Autodesk Inventor part; units mm, degrees
ref_plane "YZ Plane" through (0, 0, 0) normal (1, 0, 0) x (0, 1, 0)
ref_plane "XZ Plane" through (0, 0, 0) normal (0, 1, 0) x (-1, 0, 0)
ref_plane "XY Plane" through (0, 0, 0) normal (0, 0, 1) x (1, 0, 0)
sketch "Sketch1" plane through (0, 0, 0) normal (0, 0, 1) x (1, 0, 0)
  line L0 (0, 0) -> (861.06, 0)
  line L1 (861.06, 0) -> (861.06, 160.02)
  line L2 (861.06, 160.02) -> (0, 160.02)
  line L3 (0, 160.02) -> (0, 0)
  dimension "d2" = 861.06
  dimension "d3" = 160.02
extrude "Extrusion1" add sketch "Sketch1" along normal blind 4.7625
sketch "Sketch2" plane through (0, 0, 4.7625) normal (0, 0, 1) x (1, 0, 0)
  line L0 (849.63, 151.0147) -> (11.43, 151.0147)
  line L1 (887.73, 10.6797) -> (-26.67, 10.6797)
  line L2 (849.63, 848.8797) -> (849.63, 10.6797)
  line L3 (11.43, 848.8797) -> (11.43, 10.6797)
  line L4 (849.63, 10.6797) -> (11.43, 10.6797)
  line L5 (11.43, 10.6797) -> (11.43, 151.0147)
  line L6 (11.43, 151.0147) -> (849.63, 151.0147)
  line L7 (849.63, 151.0147) -> (849.63, 10.6797)
  point P0 (0, 0)
extrude "Extrusion2" add sketch "Sketch2" along normal blind 25.4
properties part number "gatorboard_01875in_front_door"
Work out the finished part from the listing and answer in its coordinate system (mm). A direction names the side the tool comes from. Give positions to 0.01 mm unless a question says otherwise; leave off trailing zeros. Loops run counter-clockwise (first coordinate to the right, second up) from the corner with the lowest first, then second, coordinate; pieces in that order, holes last. Notation, with made-up numbers: (-27.75, 69.25) - (-1.75, 69.25) arc R17 ccw to (-1.75, 97.25) - close; hole circle Ø5 at (-1, -30.75). An arc over 180 degrees is marked (long way). Answer in a Markdown table with one row per item. Add a question column.
Q1. Consider line 1 along Y through (x, z) = (387.5, 19.5); line 2 along X through (y, z) = (32.5, 9); line 3 along Z through (x, y) = (444, 152.5). Determine where each line is inside the solid, lowest interval first.
Q2. The part is cut by section A-A (y = 84.5). Determine the outline of the cut face in (x, z), and give its area (3 significant figures).
Q3. A tool of negligible diameter and unlimited length cuts with its end or side. For faces 1 (the flat face through (11.43, 82, 17)), 2 (the flat face through (436, 10.68, 17)), 3 (the flat face through (436, 151.015, 17)), 4 (the flat face through (425, 81, 0)), 5 (the flat face through (849.63, 82, 17)), from which of +Z, -Z, +X, -X, +Y, -Y can it reach the whole face along a straight path? Write none if from no direction.
Q4. Each of these flat-tipped pins is pushed along its axis until it touches: P1, Ø4, axis at x = 362, y = 109.5, coming from the -Z side; P2, Ø5, axis at y = 63.5, z = 12.5, coming from the +X side; P3, Ø7.5, axis at x = 314.5, z = 16.5, coming from the +Y side; P4, Ø3, axis at y = 105.5, z = 10, coming from the -X side. Where does it stop, or does it pass through?
Q5. The part is cut by section C-C (z = 24). Determine the outline of the cut face in (x, y).
Q6. The part is cut by section B-B (x = 771.5). Determine the outline of the cut face in (y, z), and give its area (3 significant figures).
Solution:
| question | item | result |
|---|---|---|
| 1 | line 1 | y = 10.68 to 151.01 |
| 1 | line 2 | x = 11.43 to 849.63 |
| 1 | line 3 | z = 0 to 4.76 |
| 2 | outline | (0, 0) - (861.06, 0) - (861.06, 4.76) - (849.63, 4.76) - (849.63, 30.16) - (11.43, 30.16) - (11.43, 4.76) - (0, 4.76) - close |
| 2 | area | 25,400 mm² |
| 3 | face 1 | +Z, -X, +Y, -Y |
| 3 | face 2 | +Z, +X, -X, -Y |
| 3 | face 3 | +Z, +X, -X, +Y |
| 3 | face 4 | -Z, +X, -X, +Y, -Y |
| 3 | face 5 | +Z, +X, +Y, -Y |
| 4 | P1 | stops at z = 0 |
| 4 | P2 | stops at x = 849.63 |
| 4 | P3 | stops at y = 151.01 |
| 4 | P4 | stops at x = 11.43 |
| 5 | outline | (11.43, 10.68) - (849.63, 10.68) - (849.63, 151.01) - (11.43, 151.01) - close |
| 6 | outline | (0, 0) - (160.02, 0) - (160.02, 4.76) - (151.01, 4.76) - (151.01, 30.16) - (10.68, 30.16) - (10.68, 4.76) - (0, 4.76) - close |
| 6 | area | 4,330 mm² |
